Check sheet for the modelled part. Datum: model origin and axes. Units: mm. A direction names the side the tool comes from. Give positions to 0.01 mm unless a question says otherwise; leave off trailing zeros. Order: outer loops, then holes, each group sorted by start corner. A loop starts at its lowest first (then second) coordinate and runs counter-clockwise, first axis right, second up.
from build123d import *

# Parameters (mm, degrees)
BOSS_EXTRUDE1_DEPTH = 6.35
SKETCH3_R           = 9.525
SKETCH3_R_2         = 2
SKETCH3_R_3         = 2.38125
CUT_EXTRUDE1_DEPTH  = 6.35
SKETCH4_W           = 17.145
SKETCH4_H           = 6.35
BOSS_EXTRUDE2_DEPTH = 4.7625
SKETCH5_W           = 6.35
SKETCH5_H           = 12.065
BOSS_EXTRUDE3_DEPTH = 4.7625
SKETCH6_W           = 6.35
SKETCH6_H           = 12.065
BOSS_EXTRUDE4_DEPTH = 4.7625
SKETCH7_W           = 12.7
SKETCH7_H           = 6.35
BOSS_EXTRUDE5_DEPTH = 4.7625


with BuildPart() as part:
    # Sketch2 → Boss-Extrude1 (new body)
    with BuildSketch(Plane.XY):
        Polygon((24.384, 80.772), (-24.384, 80.772), (-63.652178597, 13.109189138), (-55.88, 0), (55.88, 0), (63.652178597, 13.109189138), align=None)
    extrude(amount=BOSS_EXTRUDE1_DEPTH)

    # Sketch3 → Cut-Extrude1 (cut)
    with BuildSketch(Plane.XY.offset(6.35)):
        with Locations((0, 38.1)):
            Circle(SKETCH3_R)
        with Locations((-11.313708499, 49.413708499)):
            Circle(SKETCH3_R_2)
        with Locations((-11.313708499, 26.786291501)):
            Circle(SKETCH3_R_2)
        with Locations((11.313708499, 26.786291501)):
            Circle(SKETCH3_R_2)
        with Locations((11.313708499, 49.413708499)):
            Circle(SKETCH3_R_2)
        with Locations((26.516504294, 64.616504294)):
            Circle(SKETCH3_R_2)
        with Locations((-26.516504294, 64.616504294)):
            Circle(SKETCH3_R_2)
        with Locations((-26.516504294, 11.583495706)):
            Circle(SKETCH3_R_2)
        with Locations((26.516504294, 11.583495706)):
            Circle(SKETCH3_R_2)
        with Locations((0, 70.612)):
            Circle(SKETCH3_R_3)
    extrude(amount=-CUT_EXTRUDE1_DEPTH, mode=Mode.SUBTRACT)

    # Sketch4 → Boss-Extrude2 (add)
    with BuildSketch(Plane.XZ):
        with Locations((0, 3.175)):
            Rectangle(SKETCH4_W, SKETCH4_H)
    extrude(amount=BOSS_EXTRUDE2_DEPTH)

    # Sketch5 → Boss-Extrude3 (add)
    with BuildSketch(Plane(origin=(-53.306195658, 30.936302893, 0), x_dir=(0, 0, 1), z_dir=(-0.8648994127942479, 0.5019452218600805, 0))):
        with Locations((3.175, 18.75822308)):
            Rectangle(SKETCH5_W, SKETCH5_H)
    extrude(amount=BOSS_EXTRUDE3_DEPTH)

    # Sketch6 → Boss-Extrude4 (add)
    with BuildSketch(Plane(origin=(53.306195658, 30.936302893, 0), x_dir=(0, 0, -1), z_dir=(0.8648994127942479, 0.5019452218600805, 0))):
        with Locations((-3.175, 18.75822308)):
            Rectangle(SKETCH6_W, SKETCH6_H)
    extrude(amount=BOSS_EXTRUDE4_DEPTH)

    # Sketch7 → Boss-Extrude5 (add)
    with BuildSketch(Plane(origin=(0, 80.772, 0), x_dir=(1, 0, 0), z_dir=(0, 1, 0))):
        with Locations((0, -3.175)):
            Rectangle(SKETCH7_W, SKETCH7_H)
    extrude(amount=BOSS_EXTRUDE5_DEPTH)


solid = part.part
1) Section check A-A, the plane x = 0. State how many separate pieces and enclosed holes the cut face has, then the cut area to 3 significant figures.
Recorded:
separate pieces: 3
enclosed holes: 0
area: 422 mm2
2) Depth check by flat-ended pin: pin 1 Ø7.5 at (x, y) = (0, 70.612) entering from +Z; pin 2 Ø2.5 at (y, z) = (-1.5, 4.5) entering from +X; pin 3 Ø1.5 at (x, z) = (-47, 5.5) entering from -Y. Enter the tip coordinate at first touch or a pass-through.
Recorded:
pin 1: stops at z = 6.35
pin 2: stops at x = 8.57
pin 3: stops at y = 0
3) Section check B-B, the plane y = 38.1. Record the cut outline in (x, z) (3 decimals).
Recorded:
outline: (-49.149, 0) - (-9.525, 0) - (-9.525, 6.35) - (-49.149, 6.35) - close; (9.525, 0) - (49.149, 0) - (49.149, 6.35) - (9.525, 6.35) - close
4) Section check D-D, the plane x = 26. Record the cut outline in (y, z).
Recorded:
outline: (0, 0) - (9.65, 0) - (9.65, 6.35) - (0, 6.35) - close; (13.52, 0) - (62.68, 0) - (62.68, 6.35) - (13.52, 6.35) - close; (66.55, 0) - (77.99, 0) - (77.99, 6.35) - (66.55, 6.35) - close
5) Material ranges on L1, parallel to Y at x = -22.5, z = 1.75; L2, parallel to Y at x = 26, z = 4; L3, parallel to Y at x = -26.5, z = 4, recorded low to high.
Recorded:
L1: y = 0 to 80.77
L2: y = 0 to 9.65, 13.52 to 62.68, 66.55 to 77.99
L3: y = 0 to 9.58, 13.58 to 62.62, 66.62 to 77.13
6) Draft check along Y on faces 1 (the face through (-28.515, 64.704, 3.219)), 2 (the face through (-6.35, 83, 3)), 3 (the face through (0, 85.535, 3)). Enter one of: +Y half, -Y half, draft (parallel to the pull), parting line (faces both ways), or undercut.
Recorded:
face 1: undercut
face 2: draft
face 3: +Y half
7) Set-up check for faces 4 (the face through (-15, 80.772, 3)), 5 (the face through (-33, 0, 3)), 6 (the face through (48.95, 43.12, 3.22)): record each of +Z, -Z, +X, -X, +Y, -Y from which the full face is reachable in a straight line by a thin tool's end or side.
Recorded:
face 4: +Z, -Z, -X, +Y
face 5: +Z, -Z, -X, -Y
face 6: +Z, -Z, +X
